from build123d import *

# Parameters (mm, degrees)
SKETCH1_R           = 2.7
BOSS_EXTRUDE1_DEPTH = 5
SKETCH2_W           = 22.352
SKETCH2_H           = 5
BOSS_EXTRUDE2_DEPTH = 30
CUT_EXTRUDE1_DEPTH  = 5
BOSS_EXTRUDE3_DEPTH = 2
BOSS_EXTRUDE4_DEPTH = 2
SKETCH7_W           = 22.352
SKETCH7_H           = 36.907486172
BOSS_EXTRUDE5_DEPTH = 5
SKETCH8_R           = 2.7
CUT_EXTRUDE2_DEPTH  = 5
SKETCH9_W           = 22.352
SKETCH9_H           = 5
CUT_EXTRUDE3_DEPTH  = 15


with BuildPart() as part:
    # Sketch1 → Boss-Extrude1 (new body)
    with BuildSketch(Plane(origin=(0, 0, 0), x_dir=(1, 0, 0), z_dir=(0, 1, 0))):
        Polygon((0.666305019, -42.873782933), (-10.509694981, -42.873782933), (-10.509694981, -15.816806264), (-10.509694981, 42.540630423), (11.842305019, 42.540630423), (11.842305019, -42.873782933), align=None)
        with Locations(Location((0.666305019, 31.319617067, 0), (0, 0, 270))):
            Circle(SKETCH1_R, mode=Mode.SUBTRACT)
        with Locations(Location((0.666305019, 14.250817067, 0), (0, 0, 270))):
            Circle(SKETCH1_R, mode=Mode.SUBTRACT)
    extrude(amount=BOSS_EXTRUDE1_DEPTH)

    # Sketch2 → Boss-Extrude2 (add)
    with BuildSketch(Plane(origin=(0, 5, 0), x_dir=(1, 0, 0), z_dir=(0, 1, 0))):
        with Locations((0.666305019, -40.373782933)):
            Rectangle(SKETCH2_W, SKETCH2_H)
    extrude(amount=BOSS_EXTRUDE2_DEPTH)

    # Sketch3 → Cut-Extrude1 (cut)
    with BuildSketch(Plane(origin=(0, 0, 37.873782933), x_dir=(-1, 0, 0), z_dir=(0, 0, -1))):
        with BuildLine():
            Line((-2.666305019, 20), (-2.666305019, 15))
            ThreePointArc((-2.666305019, 15), (-0.666305019, 13), (1.333694981, 15))
            Line((1.333694981, 15), (1.333694981, 20))
            ThreePointArc((1.333694981, 20), (-0.666305019, 22), (-2.666305019, 20))
        make_face()
    extrude(amount=-CUT_EXTRUDE1_DEPTH, mode=Mode.SUBTRACT)

    # Sketch4 → Boss-Extrude3 (add)
    with BuildSketch(Plane(origin=(11.842305019, 0, 0), x_dir=(0, 0, -1), z_dir=(1, 0, 0))):
        Polygon((-37.873782933, 35), (-37.873782933, 5), (-7.873782933, 5), align=None)
    extrude(amount=-BOSS_EXTRUDE3_DEPTH)

    # Sketch5 → Boss-Extrude4 (add)
    with BuildSketch(Plane.ZY.offset(10.509694981)):
        Polygon((37.873782933, 35), (7.873782933, 5), (37.873782933, 5), align=None)
    extrude(amount=-BOSS_EXTRUDE4_DEPTH)

    # Sketch7 → Boss-Extrude5 (add)
    with BuildSketch(Plane.XZ):
        with Locations((0.666305019, -24.086887337)):
            Rectangle(SKETCH7_W, SKETCH7_H)
    extrude(amount=-BOSS_EXTRUDE5_DEPTH)

    # Sketch8 → Cut-Extrude2 (cut)
    with BuildSketch(Plane.XZ):
        with Locations(Location((0.666305019, -0.826217067, 0), (0, 0, 270))):
            Circle(SKETCH8_R)
        with Locations(Location((0.666305019, -18.326217067, 0), (0, 0, 270))):
            Circle(SKETCH8_R)
    extrude(amount=-CUT_EXTRUDE2_DEPTH, mode=Mode.SUBTRACT)

    # Sketch9 → Cut-Extrude3 (cut)
    with BuildSketch(Plane(origin=(0, 0, -42.540630423), x_dir=(-1, 0, 0), z_dir=(0, 0, -1))):
        with Locations((-0.666305019, 2.5)):
            Rectangle(SKETCH9_W, SKETCH9_H)
    extrude(amount=-CUT_EXTRUDE3_DEPTH, mode=Mode.SUBTRACT)


solid = part.part
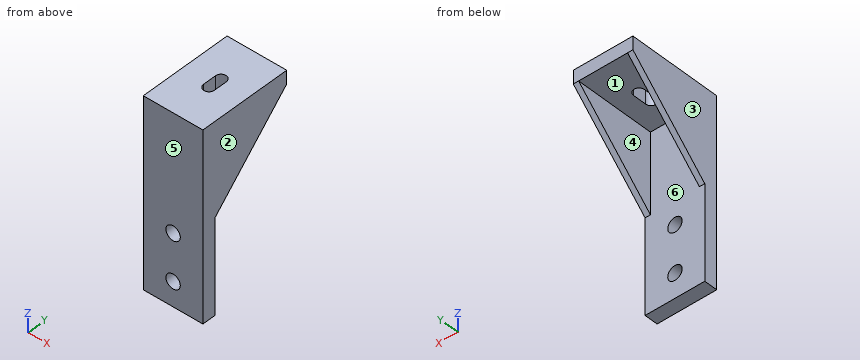
Work out the finished part from the listing and answer in its coordinate system (mm). Face numbers are marked on the shaded views. A direction names the side the tool comes from. Give positions to 0.01 mm unless a question says otherwise; leave off trailing zeros. Loops run counter-clockwise (first coordinate to the right, second up) from the corner with the lowest first, then second, coordinate; pieces in that order, holes last. Notation, with made-up numbers: (9.5, 82.5) -> (68.5, 82.5) arc R19 cw to (68.5, 112.5) -> close; hole circle Ø3 at (86, 37.25). An arc over 180 degrees is marked (long way). Use a Markdown table: item, result. Add a question column.
1. For the marked faces 5 and 6, determine the directions among +Z, -Z, +X, -X, +Y, -Y from which every point of the face is accessible in a straight line to the end or side of a thin tool.
2. Find the intervals of material crossed by probe 1 along X at (y, z) = (23, 33); probe 2 along Z at (x, y) = (-1, 1); probe 3 along Y at (x, z) = (7.5, 2), in increasing order.
3. Section C-C on y = 12 is taken. Determine the outline of the cut face in (x, z).
4. Flat-ended cylindrical pins translate along their axes: pin 1 Ø3 at (x, z) = (4.5, -16) entering from +Y; pin 2 Ø8 at (x, z) = (6.5, 29) entering from +Y. Find the tip coordinate at first contact, or state that the pin passes through.
5. Determine the mould class of the marked faces 1, 2, 3 and 4 for opening direction X: released by +X, released by -X, zero draft, split by the parting line, or undercut.
6. Section D-D on z = 16.5 is taken. Determine the outline of the cut face in (x, y), and give its area (3 significant figures).
7. Section A-A on z = -2 is taken. Determine the outline of the cut face in (x, y), and give its area (3 significant figures).
8. Section B-B on x = -3.25 is taken. Determine the outline of the cut face in (y, z), and give its area (3 significant figures).
Results below:
| question | item | result |
|---|---|---|
| 1 | face 5 | +Z, -Z, +X, -X, -Y |
| 1 | face 6 | -Z, +Y |
| 2 | probe 1 | x = -10.51 to -8.51, 9.84 to 11.84 |
| 2 | probe 2 | z = -27.54 to -20.45, -16.2 to -2.95, 1.3 to 42.87 |
| 2 | probe 3 | y = 0 to 5 |
| 3 | outline | (-10.51, 14.87) -> (-8.51, 14.87) -> (-8.51, 37.87) -> (9.84, 37.87) -> (9.84, 14.87) -> (11.84, 14.87) -> (11.84, 42.87) -> (-10.51, 42.87) -> close |
| 4 | pin 1 | stops at y = 5 |
| 4 | pin 2 | stops at y = 28.32 |
| 5 | face 1 | undercut |
| 5 | face 2 | released by +X |
| 5 | face 3 | released by -X |
| 5 | face 4 | undercut |
| 6 | outline | (-10.51, 0) -> (11.84, 0) -> (11.84, 13.63) -> (9.84, 13.63) -> (9.84, 5) -> (-8.51, 5) -> (-8.51, 13.63) -> (-10.51, 13.63) -> close |
| 6 | area | 146 mm^2 |
| 7 | outline | (-10.51, 0) -> (-1.77, 0) -> (-1.77, 5) -> (-10.51, 5) -> close; (3.1, 0) -> (11.84, 0) -> (11.84, 5) -> (3.1, 5) -> close |
| 7 | area | 87.4 mm^2 |
| 8 | outline | (0, -27.54) -> (5, -27.54) -> (5, 37.87) -> (35, 37.87) -> (35, 42.87) -> (0, 42.87) -> close |
| 8 | area | 502 mm^2 |
